Check sheet for the modelled part. Datum: model origin and axes. Units: mm. A direction names the side the tool comes from. Coordinates: 2 decimals unless noted, no trailing zeros. Loops run counter-clockwise (first coordinate to the right, second up) from the corner with the lowest first, then second, coordinate; pieces in that order, holes last. Notation, with made-up numbers: M 62,-1.5 L 80,-1.5 A10 cw 80,7.5 Z; hole C 43.5,69.25 d10. An arc over 180 degrees is marked long. Answer in a Markdown table with one row per item. Add a question column.
```python
from build123d import *

# Parameters (mm, degrees)
DODANIE_WYCI_GNI_CIE1_DEPTH = 18
WYTNIJ_WYCI_GNI_CIE1_START  = -4
SZKIC4_R                    = 5
WYTNIJ_WYCI_GNI_CIE1_DEPTH  = 2
SZKIC5_R                    = 2
WYTNIJ_WYCI_GNI_CIE2_DEPTH  = 2.653427208
ZAOKR_GLENIE1_R             = 0.5
DODANIE_WYCI_GNI_CIE2_DEPTH = 18
WYTNIJ_WYCI_GNI_CIE3_REACH  = 13.75
SFAZOWANIE1_SIZE            = 1.5


with BuildPart() as part:
    # Szkic1 → Dodanie-wyciągnięcie1 (new body)
    with BuildSketch(Plane.XY):
        Polygon((-13.5, 3.7), (-13.5, 6.5), (13.5, 6.5), (13.5, 3.7), (8.5, 3.7), (8.5, 1.5), (16.5, 1.5), (16.5, 5.5), (35, 5.5), (35, 9.5), (-35, 9.5), (-35, 5.5), (-16.5, 5.5), (-16.5, 1.5), (-8.5, 1.5), (-8.5, 3.7), align=None)
    extrude(amount=DODANIE_WYCI_GNI_CIE1_DEPTH)

    # Szkic4 → Wytnij-wyciągnięcie1 (cut)
    with BuildSketch(Plane(origin=(0, 9.5, 0), x_dir=(1, 0, 0), z_dir=(0, 1, 0)).offset(WYTNIJ_WYCI_GNI_CIE1_START)):
        with Locations((-28, -9.5)):
            Circle(SZKIC4_R)
        with Locations((28, -9.5)):
            Circle(SZKIC4_R)
    extrude(amount=WYTNIJ_WYCI_GNI_CIE1_DEPTH, mode=Mode.SUBTRACT)

    # Szkic5 → Wytnij-wyciągnięcie2 (cut)
    with BuildSketch(Plane(origin=(0, 7.5, 0), x_dir=(-1, 0, 0), z_dir=(0, -1, 0))):
        with Locations((28, -9.5)):
            Circle(SZKIC5_R)
        with Locations((-28, -9.5)):
            Circle(SZKIC5_R)
    extrude(amount=-WYTNIJ_WYCI_GNI_CIE2_DEPTH, mode=Mode.SUBTRACT)

    # Zaokrąglenie1
    zaokr_glenie1_edges = [part.edges().sort_by_distance(p)[0] for p in [
        (-16.5, 5.5, 9),
        (16.5, 5.5, 9),
        (13.5, 6.5, 9),
        (-13.5, 6.5, 9),
    ]]
    fillet(zaokr_glenie1_edges, radius=ZAOKR_GLENIE1_R)

    # Szkic6 → Dodanie-wyciągnięcie2 (add)
    with BuildSketch(Plane.XY.offset(18)):
        with BuildLine():
            Line((35, 11), (-35, 11))
            ThreePointArc((-35, 11), (-35.75, 10.25), (-35, 9.5))
            Line((-35, 9.5), (-35, 5.5))
            Line((-35, 5.5), (-37.5, 5.5))
            Line((-37.5, 5.5), (-37.5, 13.25))
            Line((-37.5, 13.25), (37.5, 13.25))
            Line((37.5, 13.25), (37.5, 5.5))
            Line((37.5, 5.5), (35, 5.5))
            Line((35, 5.5), (35, 9.5))
            ThreePointArc((35, 9.5), (35.75, 10.25), (35, 11))
        make_face()
    extrude(amount=-DODANIE_WYCI_GNI_CIE2_DEPTH)

    # Szkic7 → Wytnij-wyciągnięcie3 (cut, up to next)
    with BuildSketch(Plane(origin=(0, 13.25, 0), x_dir=(1, 0, 0), z_dir=(0, 1, 0)), mode=Mode.PRIVATE) as wytnij_wyci_gni_cie3_sk1:
        Polygon((-31.5, -7.479274058), (-31.5, -11.520725942), (-28, -13.541451884), (-24.5, -11.520725942), (-24.5, -7.479274058), (-28, -5.458548116), align=None)
    wytnij_wyci_gni_cie3_tool1 = extrude(wytnij_wyci_gni_cie3_sk1.sketch, amount=-WYTNIJ_WYCI_GNI_CIE3_REACH, mode=Mode.PRIVATE) & part.part
    add(wytnij_wyci_gni_cie3_tool1.solids().sort_by_distance((-28, 13.25, 9.5))[0], mode=Mode.SUBTRACT)
    # Szkic7 → Wytnij-wyciągnięcie3 (cut, up to next)
    with BuildSketch(Plane(origin=(0, 13.25, 0), x_dir=(1, 0, 0), z_dir=(0, 1, 0)), mode=Mode.PRIVATE) as wytnij_wyci_gni_cie3_sk2:
        Polygon((28, -5.458548116), (24.5, -7.479274058), (24.5, -11.520725942), (28, -13.541451884), (31.5, -11.520725942), (31.5, -7.479274058), align=None)
    wytnij_wyci_gni_cie3_tool2 = extrude(wytnij_wyci_gni_cie3_sk2.sketch, amount=-WYTNIJ_WYCI_GNI_CIE3_REACH, mode=Mode.PRIVATE) & part.part
    add(wytnij_wyci_gni_cie3_tool2.solids().sort_by_distance((28, 13.25, 9.5))[0], mode=Mode.SUBTRACT)

    # Sfazowanie1
    sfazowanie1_edges = [part.edges().sort_by_distance(p)[0] for p in [
        (-8.5, 2.6, 0),
        (8.5, 2.6, 0),
        (11, 3.7, 0),
        (-13.5, 4.85, 0),
        (-11, 3.7, 0),
        (0, 6.5, 0),
        (13.5, 4.85, 0),
        (-13.353553391, 6.353553391, 0),
        (13.353553391, 6.353553391, 0),
    ]]
    chamfer(sfazowanie1_edges, length=SFAZOWANIE1_SIZE)


solid = part.part
```
Q1. Cross-section at A-A (x = 11.5). Record the cut outline in (y, z), plus the area to 3 significant figures.
Q2. Mould release check, pull along Y, two halves, no side actions. Record for faces 1 (the face through (12, 1.5, 9)), 2 (the face through (11, 3.7, 10)), 3 (the face through (0, 6.5, 10)), 4 (the face through (29.726, 12.141, 12.545)): released by +Y, released by -Y, zero draft, split by the parting line, or undercut.
Q3. Cross-section at B-B (y = 10.25). Record the cut outline in (x, z), plus the area to 3 significant figures.
Q4. Cross-section at D-D (z = 9.5). Count the separate pieces of the cut face and the enclosed holes in it, plus the area to 3 significant figures.
Q5. Go/stop test with flat-tipped pins: pin 1 (1.8 mm diameter, centred on y = 2.5, z = 11, fed in from -X); pin 2 (3 mm diameter, centred on y = 3, z = 6, fed in from +X); pin 3 (1.8 mm diameter, centred on y = 5, z = 13.5, fed in from +X); pin 4 (2.5 mm diameter, centred on x = -28, z = 9.5, fed in from -Y). Record where each tip stops, or that it passes through.
Q6. Cross-section at C-C (x = 1). Record the cut outline in (y, z), plus the area to 3 significant figures.
Q7. Thickness scan on L1, parallel to X at y = 8.9, z = 9.5; L2, parallel to Y at x = -25, z = 1.5; L3, parallel to X at y = 10.25, z = 12. Record the ranges inside material, lowest first.
Q8. Access from +Z, -Z, +X, -X, +Y, -Y to the whole of each face (thin tool, end or side, straight path). Record for faces 5 (the face through (-32.995, 6.486, 9.28)), 6 (the face through (31.5, 12, 10)), 7 (the face through (9, 2, 1)), 8 (the face through (0, 11, 9)), 9 (the face through (-8.5, 3, 10)).
Answer key:
| question | item | result |
|---|---|---|
| 1 | outline | M 1.5,0 L 2.2,0 L 3.7,1.5 L 3.7,18 L 1.5,18 Z; M 6.5,1.5 L 8,0 L 9.5,0 L 9.5,18 L 6.5,18 Z; M 11,0 L 13.25,0 L 13.25,18 L 11,18 Z |
| 1 | area | 132 mm^2 |
| 2 | face 1 | released by -Y |
| 2 | face 2 | undercut |
| 2 | face 3 | undercut |
| 2 | face 4 | zero draft |
| 3 | outline | M -37.5,0 L -35.75,0 L -35.75,18 L -37.5,18 Z; M 35.75,0 L 37.5,0 L 37.5,18 L 35.75,18 Z |
| 3 | area | 63.0 mm^2 |
| 4 | separate pieces | 4 |
| 4 | enclosed holes | 0 |
| 4 | area | 406 mm^2 |
| 5 | pin 1 | x = -16.5 |
| 5 | pin 2 | x = 16.5 |
| 5 | pin 3 | x = 37.5 |
| 5 | pin 4 | through |
| 6 | outline | M 6.5,1.5 L 8,0 L 9.5,0 L 9.5,18 L 6.5,18 Z; M 11,0 L 13.25,0 L 13.25,18 L 11,18 Z |
| 6 | area | 93.4 mm^2 |
| 7 | L1 | -37.5 to -30, -26 to 26, 30 to 37.5 |
| 7 | L2 | 5.5 to 9.5, 11 to 13.25 |
| 7 | L3 | -37.5 to -35.75, 35.75 to 37.5 |
| 8 | face 5 | -Y |
| 8 | face 6 | +Y |
| 8 | face 7 | -Z, -Y |
| 8 | face 8 | +Z, -Z |
| 8 | face 9 | +Z, -Z, -Y |
